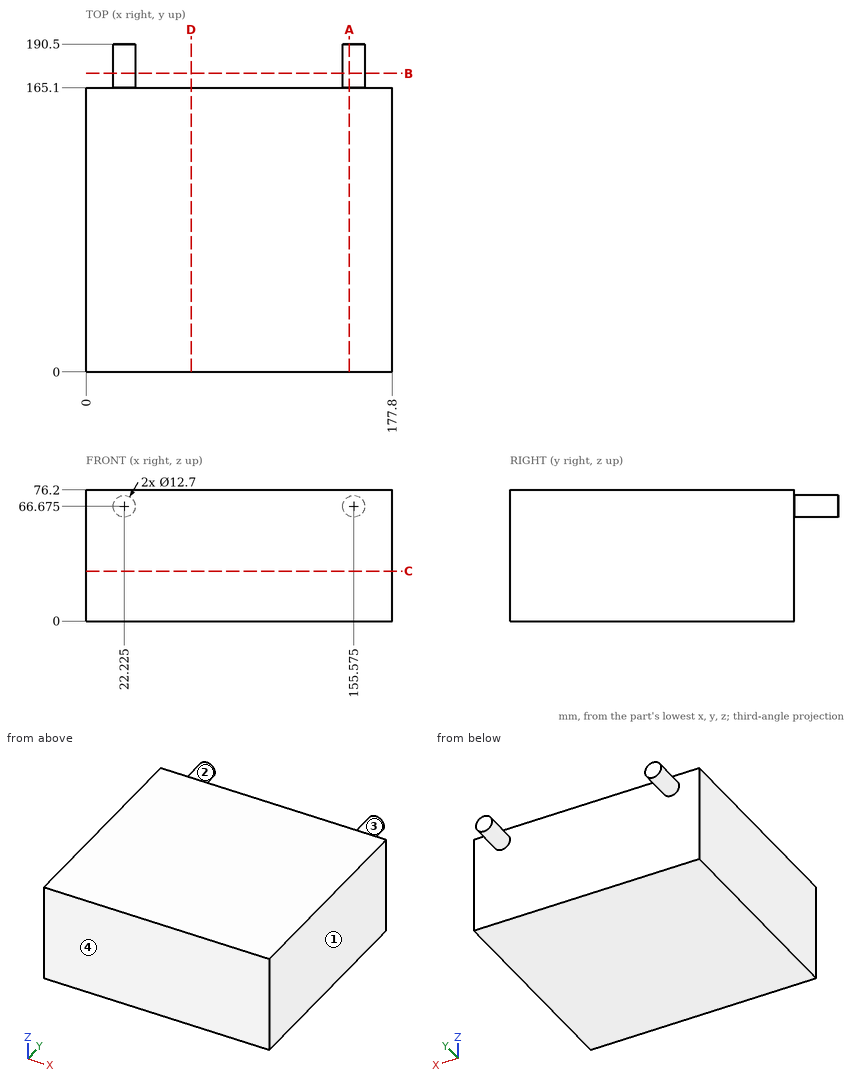
Design review of the part shown in the three views and the two pictorial views. Dimensions are in mm from the part's minimum x, y and z. Round coordinates to 2 decimals unless told otherwise and drop trailing zeros. Write each loop counter-clockwise with the first axis right and the second up, starting at its lowest first coordinate (ties: lowest second). Pieces come first, ordered by that corner, then holes. Notation, with made-up numbers: M -13,48 L 14,48 A30 ccw 14,87 Z; hole C 81,23.25 d7. An arc over 180 degrees is marked long. One line per item, written item: value. Start each with the question number.
1. Take a section at A-A on x = 153. State the section outline as (y, z) points.
2. Draft analysis for pull direction X (two halves, no side actions). For the marked faces 1, 2, 3 and 4, state which applies: pulls with the +X half, pulls with the -X half, needs draft (parallel to the pull), parting line crosses it, or undercut.
3. To check wall thickness, follow probe 1 along Y at (x, z) = (52, 6); probe 2 along X at (y, z) = (178, 64); probe 3 along X at (y, z) = (173, 62). State the ranges of each line that lie inside material, in increasing order. Write a range as from..to.
4. Take a section at C-C on z = 29. State the section outline as (x, y) points.
5. Take a section at D-D on x = 61. State the section outline as (y, z) points.
6. Take a section at B-B on y = 173.5. State the section outline as (x, z) points (3 decimals).
7. Clearance check with flat-ended pins moving along their axes: P1, Ø12, axis at x = 63, y = 35.5, coming from the -Z side; P2, Ø1.5, axis at x = 51.5, z = 60, coming from the +Y side. State where each tip first meets the part, or that it passes through.
Computed:
1. outline: M 0,0 L 165.1,0 L 165.1,60.87 L 190.5,60.87 L 190.5,72.48 L 165.1,72.48 L 165.1,76.2 L 0,76.2 Z
2. face 1: pulls with the +X half
2. face 2: undercut
2. face 3: undercut
2. face 4: needs draft
3. probe 1: y = 0..165.1
3. probe 2: x = 16.47..27.98, 149.82..161.33
3. probe 3: x = 17.93..26.52, 151.28..159.87
4. outline: M 0,0 L 177.8,0 L 177.8,165.1 L 0,165.1 Z
5. outline: M 0,0 L 165.1,0 L 165.1,76.2 L 0,76.2 Z
6. outline: C 22.225,66.675 d12.7; C 155.575,66.675 d12.7
7. P1: stops at z = 0
7. P2: stops at y = 165.1
